For this review, take the finished solid that the model builds, in its own axes (mm). Round coordinates to 2 decimals unless told otherwise and drop trailing zeros. Order: outer loops, then holes, each group sorted by start corner. A loop starts at its lowest first (then second) coordinate and runs counter-clockwise, first axis right, second up. Notation, with made-up numbers: (20.25, 60) - (68.25, 60) arc R27 ccw to (68.25, 93) - close; hole circle Ø6 at (-18, -39). An arc over 180 degrees is marked (long way). One line per item, written item: value.
```python
from build123d import *

# Parameters (mm, degrees)
BOSS_EXTRUDE1_DEPTH = 3
CUT_EXTRUDE1_REACH  = 91.591
SKETCH2_R           = 3
SKETCH2_W           = 7
SKETCH2_H           = 55
SKETCH2_W_2         = 2.5
SKETCH2_H_2         = 40
SKETCH2_H_3         = 10
SKETCH2_W_3         = 5
SKETCH2_H_4         = 2.5
SKETCH2_W_4         = 8
SKETCH2_W_5         = 10
SKETCH2_H_5         = 16
SKETCH2_W_6         = 15
SKETCH2_H_6         = 17


with BuildPart() as part:
    # Sketch1 → Boss-Extrude1 (new body)
    with BuildSketch(Plane.XY):
        with BuildLine():
            Line((40, 40.219178082), (-40, 40.219178082))
            ThreePointArc((-40, 40.219178082), (-80, 0.219178082), (-40, -39.780821918))
            Line((-40, -39.780821918), (40, -39.780821918))
            ThreePointArc((40, -39.780821918), (80, 0.219178082), (40, 40.219178082))
        make_face()
    extrude(amount=BOSS_EXTRUDE1_DEPTH)

    # Sketch2 → Cut-Extrude1 (cut, up to next)
    with BuildSketch(Plane(origin=(0, 0, 0), x_dir=(-1, 0, 0), z_dir=(0, 0, -1)), mode=Mode.PRIVATE) as cut_extrude1_sk1:
        with Locations((-35, 32.219178082)):
            Circle(SKETCH2_R)
    cut_extrude1_tool1 = extrude(cut_extrude1_sk1.sketch, amount=-CUT_EXTRUDE1_REACH, mode=Mode.PRIVATE) & part.part
    # Sketch2 → Cut-Extrude1 (cut, up to next)
    with BuildSketch(Plane(origin=(0, 0, 0), x_dir=(-1, 0, 0), z_dir=(0, 0, -1)), mode=Mode.PRIVATE) as cut_extrude1_sk2:
        with Locations((-35, -31.780821918)):
            Circle(SKETCH2_R)
    cut_extrude1_tool2 = extrude(cut_extrude1_sk2.sketch, amount=-CUT_EXTRUDE1_REACH, mode=Mode.PRIVATE) & part.part
    # Sketch2 → Cut-Extrude1 (cut, up to next)
    with BuildSketch(Plane(origin=(0, 0, 0), x_dir=(-1, 0, 0), z_dir=(0, 0, -1)), mode=Mode.PRIVATE) as cut_extrude1_sk3:
        with Locations((35, 32.219178082)):
            Circle(SKETCH2_R)
    cut_extrude1_tool3 = extrude(cut_extrude1_sk3.sketch, amount=-CUT_EXTRUDE1_REACH, mode=Mode.PRIVATE) & part.part
    # Sketch2 → Cut-Extrude1 (cut, up to next)
    with BuildSketch(Plane(origin=(0, 0, 0), x_dir=(-1, 0, 0), z_dir=(0, 0, -1)), mode=Mode.PRIVATE) as cut_extrude1_sk4:
        with Locations((35, -31.780821918)):
            Circle(SKETCH2_R)
    cut_extrude1_tool4 = extrude(cut_extrude1_sk4.sketch, amount=-CUT_EXTRUDE1_REACH, mode=Mode.PRIVATE) & part.part
    # Sketch2 → Cut-Extrude1 (cut, up to next)
    with BuildSketch(Plane(origin=(0, 0, 0), x_dir=(-1, 0, 0), z_dir=(0, 0, -1)), mode=Mode.PRIVATE) as cut_extrude1_sk5:
        with Locations((26.5, 0)):
            Rectangle(SKETCH2_W, SKETCH2_H)
    cut_extrude1_tool5 = extrude(cut_extrude1_sk5.sketch, amount=-CUT_EXTRUDE1_REACH, mode=Mode.PRIVATE) & part.part
    # Sketch2 → Cut-Extrude1 (cut, up to next)
    with BuildSketch(Plane(origin=(0, 0, 0), x_dir=(-1, 0, 0), z_dir=(0, 0, -1)), mode=Mode.PRIVATE) as cut_extrude1_sk6:
        with Locations((-46.25, 0)):
            Rectangle(SKETCH2_W_2, SKETCH2_H_2)
    cut_extrude1_tool6 = extrude(cut_extrude1_sk6.sketch, amount=-CUT_EXTRUDE1_REACH, mode=Mode.PRIVATE) & part.part
    # Sketch2 → Cut-Extrude1 (cut, up to next)
    with BuildSketch(Plane(origin=(0, 0, 0), x_dir=(-1, 0, 0), z_dir=(0, 0, -1)), mode=Mode.PRIVATE) as cut_extrude1_sk7:
        with Locations((-46.25, 30.219178082)):
            Rectangle(SKETCH2_W_2, SKETCH2_H_3)
    cut_extrude1_tool7 = extrude(cut_extrude1_sk7.sketch, amount=-CUT_EXTRUDE1_REACH, mode=Mode.PRIVATE) & part.part
    # Sketch2 → Cut-Extrude1 (cut, up to next)
    with BuildSketch(Plane(origin=(0, 0, 0), x_dir=(-1, 0, 0), z_dir=(0, 0, -1)), mode=Mode.PRIVATE) as cut_extrude1_sk8:
        with Locations((-46.25, -29.780821918)):
            Rectangle(SKETCH2_W_2, SKETCH2_H_3)
    cut_extrude1_tool8 = extrude(cut_extrude1_sk8.sketch, amount=-CUT_EXTRUDE1_REACH, mode=Mode.PRIVATE) & part.part
    # Sketch2 → Cut-Extrude1 (cut, up to next)
    with BuildSketch(Plane(origin=(0, 0, 0), x_dir=(-1, 0, 0), z_dir=(0, 0, -1)), mode=Mode.PRIVATE) as cut_extrude1_sk9:
        with Locations((27.5, 33.969178082)):
            Rectangle(SKETCH2_W_3, SKETCH2_H_4)
    cut_extrude1_tool9 = extrude(cut_extrude1_sk9.sketch, amount=-CUT_EXTRUDE1_REACH, mode=Mode.PRIVATE) & part.part
    # Sketch2 → Cut-Extrude1 (cut, up to next)
    with BuildSketch(Plane(origin=(0, 0, 0), x_dir=(-1, 0, 0), z_dir=(0, 0, -1)), mode=Mode.PRIVATE) as cut_extrude1_sk10:
        with Locations((27.5, -33.530821918)):
            Rectangle(SKETCH2_W_3, SKETCH2_H_4)
    cut_extrude1_tool10 = extrude(cut_extrude1_sk10.sketch, amount=-CUT_EXTRUDE1_REACH, mode=Mode.PRIVATE) & part.part
    # Sketch2 → Cut-Extrude1 (cut, up to next)
    with BuildSketch(Plane(origin=(0, 0, 0), x_dir=(-1, 0, 0), z_dir=(0, 0, -1)), mode=Mode.PRIVATE) as cut_extrude1_sk11:
        with Locations((-25.5, 33.969178082)):
            Rectangle(SKETCH2_W_3, SKETCH2_H_4)
    cut_extrude1_tool11 = extrude(cut_extrude1_sk11.sketch, amount=-CUT_EXTRUDE1_REACH, mode=Mode.PRIVATE) & part.part
    # Sketch2 → Cut-Extrude1 (cut, up to next)
    with BuildSketch(Plane(origin=(0, 0, 0), x_dir=(-1, 0, 0), z_dir=(0, 0, -1)), mode=Mode.PRIVATE) as cut_extrude1_sk12:
        with Locations((-9, 33.969178082)):
            Rectangle(SKETCH2_W_4, SKETCH2_H_4)
    cut_extrude1_tool12 = extrude(cut_extrude1_sk12.sketch, amount=-CUT_EXTRUDE1_REACH, mode=Mode.PRIVATE) & part.part
    # Sketch2 → Cut-Extrude1 (cut, up to next)
    with BuildSketch(Plane(origin=(0, 0, 0), x_dir=(-1, 0, 0), z_dir=(0, 0, -1)), mode=Mode.PRIVATE) as cut_extrude1_sk13:
        with Locations((10, 33.969178082)):
            Rectangle(SKETCH2_W_5, SKETCH2_H_4)
    cut_extrude1_tool13 = extrude(cut_extrude1_sk13.sketch, amount=-CUT_EXTRUDE1_REACH, mode=Mode.PRIVATE) & part.part
    # Sketch2 → Cut-Extrude1 (cut, up to next)
    with BuildSketch(Plane(origin=(0, 0, 0), x_dir=(-1, 0, 0), z_dir=(0, 0, -1)), mode=Mode.PRIVATE) as cut_extrude1_sk14:
        with Locations((-25.5, -33.530821918)):
            Rectangle(SKETCH2_W_3, SKETCH2_H_4)
    cut_extrude1_tool14 = extrude(cut_extrude1_sk14.sketch, amount=-CUT_EXTRUDE1_REACH, mode=Mode.PRIVATE) & part.part
    # Sketch2 → Cut-Extrude1 (cut, up to next)
    with BuildSketch(Plane(origin=(0, 0, 0), x_dir=(-1, 0, 0), z_dir=(0, 0, -1)), mode=Mode.PRIVATE) as cut_extrude1_sk15:
        with Locations((-9, -33.530821918)):
            Rectangle(SKETCH2_W_4, SKETCH2_H_4)
    cut_extrude1_tool15 = extrude(cut_extrude1_sk15.sketch, amount=-CUT_EXTRUDE1_REACH, mode=Mode.PRIVATE) & part.part
    # Sketch2 → Cut-Extrude1 (cut, up to next)
    with BuildSketch(Plane(origin=(0, 0, 0), x_dir=(-1, 0, 0), z_dir=(0, 0, -1)), mode=Mode.PRIVATE) as cut_extrude1_sk16:
        with Locations((10, -33.530821918)):
            Rectangle(SKETCH2_W_5, SKETCH2_H_4)
    cut_extrude1_tool16 = extrude(cut_extrude1_sk16.sketch, amount=-CUT_EXTRUDE1_REACH, mode=Mode.PRIVATE) & part.part
    # Sketch2 → Cut-Extrude1 (cut, up to next)
    with BuildSketch(Plane(origin=(0, 0, 0), x_dir=(-1, 0, 0), z_dir=(0, 0, -1)), mode=Mode.PRIVATE) as cut_extrude1_sk17:
        with Locations((43.5, -18)):
            Rectangle(SKETCH2_W, SKETCH2_H_5)
    cut_extrude1_tool17 = extrude(cut_extrude1_sk17.sketch, amount=-CUT_EXTRUDE1_REACH, mode=Mode.PRIVATE) & part.part
    # Sketch2 → Cut-Extrude1 (cut, up to next)
    with BuildSketch(Plane(origin=(0, 0, 0), x_dir=(-1, 0, 0), z_dir=(0, 0, -1)), mode=Mode.PRIVATE) as cut_extrude1_sk18:
        with Locations((47.5, 18.5)):
            Rectangle(SKETCH2_W_6, SKETCH2_H_6)
    cut_extrude1_tool18 = extrude(cut_extrude1_sk18.sketch, amount=-CUT_EXTRUDE1_REACH, mode=Mode.PRIVATE) & part.part
    add(cut_extrude1_tool1.solids().sort_by_distance((35, 32.219178, 0))[0], mode=Mode.SUBTRACT)
    add(cut_extrude1_tool2.solids().sort_by_distance((35, -31.780822, 0))[0], mode=Mode.SUBTRACT)
    add(cut_extrude1_tool3.solids().sort_by_distance((-35, 32.219178, 0))[0], mode=Mode.SUBTRACT)
    add(cut_extrude1_tool4.solids().sort_by_distance((-35, -31.780822, 0))[0], mode=Mode.SUBTRACT)
    add(cut_extrude1_tool5.solids().sort_by_distance((-26.5, 0, 0))[0], mode=Mode.SUBTRACT)
    add(cut_extrude1_tool6.solids().sort_by_distance((46.25, 0, 0))[0], mode=Mode.SUBTRACT)
    add(cut_extrude1_tool7.solids().sort_by_distance((46.25, 30.219178, 0))[0], mode=Mode.SUBTRACT)
    add(cut_extrude1_tool8.solids().sort_by_distance((46.25, -29.780822, 0))[0], mode=Mode.SUBTRACT)
    add(cut_extrude1_tool9.solids().sort_by_distance((-27.5, 33.969178, 0))[0], mode=Mode.SUBTRACT)
    add(cut_extrude1_tool10.solids().sort_by_distance((-27.5, -33.530822, 0))[0], mode=Mode.SUBTRACT)
    add(cut_extrude1_tool11.solids().sort_by_distance((25.5, 33.969178, 0))[0], mode=Mode.SUBTRACT)
    add(cut_extrude1_tool12.solids().sort_by_distance((9, 33.969178, 0))[0], mode=Mode.SUBTRACT)
    add(cut_extrude1_tool13.solids().sort_by_distance((-10, 33.969178, 0))[0], mode=Mode.SUBTRACT)
    add(cut_extrude1_tool14.solids().sort_by_distance((25.5, -33.530822, 0))[0], mode=Mode.SUBTRACT)
    add(cut_extrude1_tool15.solids().sort_by_distance((9, -33.530822, 0))[0], mode=Mode.SUBTRACT)
    add(cut_extrude1_tool16.solids().sort_by_distance((-10, -33.530822, 0))[0], mode=Mode.SUBTRACT)
    add(cut_extrude1_tool17.solids().sort_by_distance((-43.5, -18, 0))[0], mode=Mode.SUBTRACT)
    add(cut_extrude1_tool18.solids().sort_by_distance((-47.5, 18.5, 0))[0], mode=Mode.SUBTRACT)


solid = part.part
```
Item 1: The part is to be moulded in two halves that separate along X. For faces 1 (the flat face through (-1, 1, 0)), 2 (the flat face through (-10, 35.219, 1)), say which applies: +X half, -X half, draft (parallel to the pull), parting line (faces both ways), or undercut.
Returned:
face 1: draft
face 2: undercut
Item 2: Take a section at D-D (y = 11.5). Write out the cut boundary in (x, z), plus the area to 3 significant figures.
Returned:
outline: (-78.38, 0) - (-55, 0) - (-55, 3) - (-78.38, 3) - close; (-40, 0) - (-30, 0) - (-30, 3) - (-40, 3) - close; (-23, 0) - (45, 0) - (45, 3) - (-23, 3) - close; (47.5, 0) - (78.38, 0) - (78.38, 3) - (47.5, 3) - close
area: 397 mm^2
Item 3: Wall thickness on line 1 (Y direction, x = -27.5, z = 1); line 2 (Y direction, x = 35, z = 1.8); line 3 (Y direction, x = 8, z = 0.75): over which ranges is each line inside the solid? List them lowest first.
Returned:
line 1: -39.78 to -34.78, -32.28 to -27.5, 27.5 to 32.72, 35.22 to 40.22
line 2: -39.78 to -34.78, -28.78 to 29.22, 35.22 to 40.22
line 3: -39.78 to -34.78, -32.28 to 32.72, 35.22 to 40.22
Item 4: Take a section at B-B (y = -1.5). Write out the cut boundary in (x, z), plus the area to 3 significant figures.
Returned:
outline: (-79.96, 0) - (-30, 0) - (-30, 3) - (-79.96, 3) - close; (-23, 0) - (45, 0) - (45, 3) - (-23, 3) - close; (47.5, 0) - (79.96, 0) - (79.96, 3) - (47.5, 3) - close
area: 451 mm^2
Item 5: Take a section at A-A (x = -35). Write out the cut boundary in (y, z), plus the area to 3 significant figures.
Returned:
outline: (-39.78, 0) - (-34.78, 0) - (-34.78, 3) - (-39.78, 3) - close; (-28.78, 0) - (29.22, 0) - (29.22, 3) - (-28.78, 3) - close; (35.22, 0) - (40.22, 0) - (40.22, 3) - (35.22, 3) - close
area: 204 mm^2
Item 6: For P1, Ø0.8, axis at y = -33, z = 1, coming from the +X side; P2, Ø1.5, axis at y = 21, z = 2, coming from the +X side; P3, Ø3.5, axis at x = -35, y = -31.78, coming from the +Z side; P4, Ø1.5, axis at y = 31, z = 1.5, coming from the -X side, all flat-tipped, find the tip position at first contact; note any pin that passes through.
Returned:
P1: x = 62.87
P2: x = 74.62
P3: through
P4: x = -66.42
Item 7: Take a section at C-C (y = -16). Write out the cut boundary in (x, z).
Returned:
outline: (-76.56, 0) - (-47, 0) - (-47, 3) - (-76.56, 3) - close; (-40, 0) - (-30, 0) - (-30, 3) - (-40, 3) - close; (-23, 0) - (45, 0) - (45, 3) - (-23, 3) - close; (47.5, 0) - (76.56, 0) - (76.56, 3) - (47.5, 3) - close
